Geometry: final body of the model. Coordinates: model frame, mm. Face numbers are marked on the shaded views. A direction names the side the tool comes from. Give positions to 0.01 mm unless a question says otherwise; leave off trailing zeros. Write each loop counter-clockwise with the first axis right and the second up, starting at its lowest first coordinate (ties: lowest second). Pieces come first, ordered by that corner, then holes. Notation, with made-up numbers: M -38,89.5 L -15,89.5 A36 cw -15,128.5 Z; hole C 52,75 d2. An arc over 180 degrees is marked long. Answer as a JSON object with one key per item and string values.
Autodesk Inventor part; units mm, degrees
ref_plane "YZ Plane" through (0, 0, 0) normal (1, 0, 0) x (0, 1, 0)
ref_plane "XZ Plane" through (0, 0, 0) normal (0, 1, 0) x (-1, 0, 0)
ref_plane "XY Plane" through (0, 0, 0) normal (0, 0, 1) x (1, 0, 0)
sketch "Sketch1" plane through (0, 0, 0) normal (0, 1, 0) x (-1, 0, 0)
  line L0 (0, 0) -> (56, 0)
  line L1 (56, 0) -> (56, -50)
  line L2 (56, -50) -> (0, -50)
  line L3 (0, -50) -> (0, 0)
  line L4 (56.2, 0) -> (-0.2, 0)
  line L5 (-0.2, 0) -> (-0.2, -50)
  line L6 (-0.2, -50) -> (56.2, -50)
  line L7 (56.2, -50) -> (56.2, 0)
  line L8 (58.7, 2.5) -> (-2.7, 2.5)
  line L9 (-2.7, 2.5) -> (-2.7, -52.5)
  line L10 (-2.7, -52.5) -> (58.7, -52.5)
  line L11 (58.7, -52.5) -> (58.7, 2.5)
  line L12 (56.2, -48.0985) -> (56.2, -52.5)
  line L13 (-0.2, -48.7936) -> (-0.2, -52.5)
  point P0 (-0.2, -50)
  dimension "d0" = 56
  dimension "d1" = 50
  dimension "d2" = 0.2
  dimension "d3" = 0.2
  dimension "d4" = 0
  dimension "d5" = 0
  dimension "d6" = 2.5
  dimension "d7" = 2.5
  dimension "d8" = 2.5
  dimension "d9" = 2.5
extrude "Extrusion1" add sketch "Sketch1" along normal blind 15.2 contours L4 L5 L13 L10 L9 L8 L11 L12 L7 L0
extrude "Extrusion2" add sketch "Sketch1" along normal blind 1
sketch "Sketch2" plane through (0.2, 15.2, 0) normal (0, 0, -1) x (-1, 0, 0)
  line L0 (0, -14.2) -> (0, 0)
  line L1 (0, -11.7) -> (56.4, -11.7)
  line L2 (56.4, -11.7) -> (56.4, -14.2)
  line L3 (56.4, -14.2) -> (0, -14.2)
  line L4 (0, -14.2) -> (0, -11.7)
  line L5 (56.4, -14.2) -> (56.4, 0)
  line L6 (0, -14.2) -> (56.4, -14.2)
  line L7 (1, -11.7) -> (55.4, -11.7)
  line L8 (55.4, -11.7) -> (55.4, -14.2)
  line L9 (55.4, -14.2) -> (1, -14.2)
  line L10 (1, -14.2) -> (1, -11.7)
  line L11 (0, -9) -> (56.4, -9)
  line L12 (56.4, -9) -> (56.4, -10)
  line L13 (56.4, -10) -> (0, -10)
  line L14 (0, -10) -> (0, -9)
  line L15 (56.4, -9) -> (55.4, -9)
  line L16 (55.4, -9) -> (55.4, -10)
  line L17 (55.4, -10) -> (56.4, -10)
  line L18 (56.4, -10) -> (56.4, -9)
  line L19 (0, -9) -> (1, -9)
  line L20 (1, -9) -> (1, -10)
  line L21 (1, -10) -> (0, -10)
  line L22 (0, -10) -> (0, -9)
  point P0 (0.2, -15.2)
  point P1 (0, -10)
  point P2 (1, -14.2)
  dimension "d14" = 0
  dimension "d16" = 2.5
  dimension "d17" = 1
  dimension "d18" = 1
  dimension "d19" = 0
  dimension "d20" = 0
  dimension "d21" = 1.7
  dimension "d22" = 1
extrude "Extrusion3" add sketch "Sketch2" along normal up to surface (52.5 mm away) contours L0 L1 L10 L3 | L0 L11 L20 L13 | L8 L1 L2 L3 | L16 L11 L5 L13
sketch "Sketch3" plane through (2.7, 0, -52.5) normal (0, 0, -1) x (-1, 0, 0)
  line L0 (2.5, 15.2) -> (58.9, 15.2)
  line L1 (23.5, 15.2) -> (43.9, 15.2)
  line L2 (43.9, 15.2) -> (43.9, 0)
  line L3 (43.9, 0) -> (23.5, 0)
  line L4 (23.5, 0) -> (23.5, 15.2)
  line L5 (58.9, 6.2) -> (58.9, 15.2)
  line L6 (2.5, 6.2) -> (2.5, 15.2)
  line L7 (0, 0) -> (61.4, 0)
  line L8 (23.5, 0) -> (43.9, 0)
  line L9 (43.9, 0) -> (43.9, 5)
  line L10 (43.9, 5) -> (23.5, 5)
  line L11 (23.5, 5) -> (23.5, 0)
  point P0 (2.7, 0)
  dimension "d25" = 15
  dimension "d26" = 21
  dimension "d27" = 0
  dimension "d30" = 5
extrude "Extrusion5" cut sketch "Sketch3" against normal blind 75.725 contours L10 L2 L3 L4
sketch "Sketch4" plane through (-58.7, 15.2, 2.5) normal (0, 0, 1) x (1, 0, 0)
  line L0 (11.5, -0.7) -> (20.5, -0.7)
  line L1 (20.5, -0.7) -> (20.5, -4.2)
  line L2 (20.5, -4.2) -> (11.5, -4.2)
  line L3 (11.5, -4.2) -> (11.5, -0.7)
  point P0 (58.7, -15.2)
  point P1 (3.5, -11.7)
  point P2 (2.5, -11.7)
  dimension "d33" = 7.5
  dimension "d34" = 11
  dimension "d35" = 18
  dimension "d36" = 9
extrude "Extrusion6" cut sketch "Sketch4" against normal up to surface (2.5 mm away)
sketch "Sketch5" plane through (0, 15.2, 0) normal (0, 1, 0) x (1, 0, 0)
  line L0 (2.7, -2.5) -> (2.7, 52.5)
  line L1 (2.7, -2.5) -> (2.7, 52.5)
  line L2 (2.7, 52.5) -> (0.2, 52.5)
  line L3 (2.7, 52.5) -> (0.2, 52.5)
  line L4 (0.2, 52.5) -> (0.2, 0)
  line L5 (0.2, 0) -> (-56.2, 0)
  line L6 (0.2, 0) -> (-56.2, 0)
  line L7 (-56.2, 52.5) -> (-58.7, 52.5)
  line L8 (-56.2, 0) -> (-56.2, 52.5)
  line L9 (-58.7, 52.5) -> (-58.7, -2.5)
  line L10 (-56.2, 52.5) -> (-58.7, 52.5)
  line L11 (-58.7, -2.5) -> (2.7, -2.5)
  line L12 (-58.7, 52.5) -> (-58.7, -2.5)
  line L13 (-58.7, -2.5) -> (2.7, -2.5)
  point P0 (0, 0)
extrude "Extrusion7" add sketch "Sketch5" along normal blind 3
sketch "Sketch6" plane through (0, 18.2, 0) normal (0, 1, 0) x (1, 0, 0)
  line L0 (2.7, -2.5) -> (2.7, 52.5)
  line L1 (-58.7, 52.5) -> (-58.7, -2.5)
  line L2 (2.7, -2.5) -> (-58.7, -2.5)
  line L3 (-58.7, -2.5) -> (-58.7, 52.5)
  line L4 (-58.7, 52.5) -> (2.7, 52.5)
  line L5 (2.7, 52.5) -> (2.7, -2.5)
  line L6 (-13.8, 42) -> (-1.8, 42)
  line L7 (-1.8, 42) -> (-1.8, 36)
  line L8 (-1.8, 36) -> (-13.8, 36)
  line L9 (-13.8, 36) -> (-13.8, 42)
  line L10 (0.2, 0) -> (-56.2, 0)
  line L11 (0.2, 52.5) -> (0.2, 0)
  line L12 (-10.8, 45) -> (-4.8, 45)
  line L13 (-13.8, 42) -> (-8.427, 47.373)
  line L14 (-13.8, 42) -> (-6.2015, 42) construction
  line L15 (-1.8, 42) -> (-7.8, 48)
  line L16 (-1.8, 42) -> (6.6853, 42) construction
  point P0 (0, 0)
  point P1 (-4.8, 45)
  point P2 (-58.7, -2.5)
  dimension "d41" = 36
  dimension "d42" = 42
  dimension "d43" = 2
  dimension "d44" = 14
  dimension "d45" = 3
  dimension "d46" = 3
  dimension "d47" = 45
  dimension "d48" = 135
  dimension "d49" = 3
extrude "Extrusion8" add sketch "Sketch6" along normal blind 1
sketch "Sketch7" plane through (2.7, 0, -52.5) normal (0, 0, -1) x (-1, 0, 0)
  line L0 (2.5, 3.5) -> (2.5, 5.2)
  line L1 (2.5, 3.5) -> (1.5, 3.5)
  line L2 (1.5, 3.5) -> (1.5, 5.2)
  line L3 (1.5, 5.2) -> (2.5, 5.2)
  line L4 (2.5, 5.2) -> (2.5, 3.5)
  line L5 (2.5, 6.2) -> (2.5, 18.2)
  line L6 (2.5, 18.2) -> (1.5, 18.2)
  line L7 (1.5, 18.2) -> (1.5, 6.2)
  line L8 (1.5, 6.2) -> (2.5, 6.2)
  line L9 (2.5, 6.2) -> (2.5, 18.2)
  line L10 (58.9, 3.5) -> (58.9, 5.2)
  line L11 (58.9, 3.5) -> (59.9, 3.5)
  line L12 (59.9, 3.5) -> (59.9, 5.2)
  line L13 (59.9, 5.2) -> (58.9, 5.2)
  line L14 (58.9, 5.2) -> (58.9, 3.5)
  line L15 (57.9, 6.2) -> (58.9, 6.2)
  line L16 (58.9, 6.2) -> (59.9, 6.2)
  line L17 (59.9, 6.2) -> (59.9, 18.2)
  line L18 (59.9, 18.2) -> (58.9, 18.2)
  line L19 (58.9, 18.2) -> (58.9, 6.2)
  point P0 (2.7, 0)
  dimension "d52" = 1
  dimension "d53" = 1
  dimension "d54" = 1
  dimension "d55" = 1
extrude "Extrusion9" cut sketch "Sketch7" against normal up to surface (52.5 mm away)
sketch "Sketch8" plane through (0, 19.2, 0) normal (0, 1, 0) x (1, 0, 0)
  line L0 (2.7, 52.5) -> (-20.8, 52.5)
  line L1 (-58.7, 52.5) -> (-58.7, -2.5)
  line L2 (2.7, 52.5) -> (-58.7, 52.5)
  line L3 (-58.7, 52.5) -> (-58.7, 49.5)
  line L4 (-58.7, 49.5) -> (2.7, 49.5)
  line L5 (2.7, 49.5) -> (2.7, 52.5)
  point P0 (0, 0)
  dimension "d58" = 3
extrude "Extrusion10" cut sketch "Sketch8" against normal up to surface (19.2 mm away)
sketch "Sketch9" plane through (0, 19.2, 0) normal (0, 1, 0) x (1, 0, 0)
  line L0 (2.7, -2.5) -> (2.7, 49.5)
  line L1 (-58.7, 49.5) -> (-58.7, -2.5)
  line L2 (2.7, 49.5) -> (-58.7, 49.5)
  line L3 (-58.7, 49.5) -> (-58.7, -2.5)
  line L4 (-58.7, -2.5) -> (2.7, -2.5)
  line L5 (2.7, -2.5) -> (2.7, 49.5)
  line L6 (-1.8, 42) -> (-1.8, 36)
  line L7 (-4.8, 45) -> (-1.8, 42)
  line L8 (-1.8, 42) -> (-4.8, 45)
  line L9 (-10.8, 45) -> (-4.8, 45)
  line L10 (-4.8, 45) -> (-10.8, 45)
  line L11 (-13.8, 42) -> (-10.8, 45)
  line L12 (-10.8, 45) -> (-13.8, 42)
  line L13 (-13.8, 36) -> (-13.8, 42)
  line L14 (-13.8, 42) -> (-13.8, 36)
  line L15 (-1.8, 36) -> (-13.8, 36)
  line L16 (-13.8, 36) -> (-1.8, 36)
  line L17 (-1.8, 36) -> (-1.8, 42)
  point P0 (0, 0)
extrude "Extrusion11" add sketch "Sketch9" along normal blind 1
sketch "Sketch10" plane through (1.2, 18.2, -49.5) normal (0, 0, -1) x (-1, 0, 0)
  line L0 (0, 0) -> (58.4, 0)
  line L1 (0, 0) -> (58.4, 0)
  line L2 (58.4, 0) -> (58.4, 1)
  line L3 (58.4, 1) -> (0, 1)
  line L4 (0, 1) -> (0, 0)
  point P0 (1.2, -18.2)
  dimension "d63" = 1
extrude "Extrusion12" cut sketch "Sketch10" against normal up to surface (49.5 mm away)
sketch "Sketch11" plane through (0, 20.2, 0) normal (0, 1, 0) x (1, 0, 0)
  line L0 (2.7, -2.5) -> (2.7, 49.5)
  line L1 (-58.7, 49.5) -> (-58.7, -2.5)
  line L2 (2.7, -2.5) -> (-58.7, -2.5)
  line L3 (-58.7, -2.5) -> (-58.7, -1)
  line L4 (-58.7, -1) -> (2.7, -1)
  line L5 (2.7, -1) -> (2.7, -2.5)
  point P0 (0, 0)
  dimension "d66" = 1.5
extrude "Extrusion13" cut sketch "Sketch11" against normal blind 24.925
sketch "Sketch12" plane through (-58.7, 20.2, 1) normal (0, 0, 1) x (1, 0, 0)
  line L0 (10.5, -3.7) -> (22.5, -3.7)
  line L1 (22.5, -3.7) -> (22.5, -11.2)
  line L2 (22.5, -11.2) -> (10.5, -11.2)
  line L3 (10.5, -11.2) -> (10.5, -3.7)
  line L4 (20.5, -5.7) -> (11.5, -5.7)
  line L5 (20.5, -9.2) -> (20.5, -5.7)
  line L6 (11.5, -9.2) -> (20.5, -9.2)
  line L7 (11.5, -5.7) -> (11.5, -9.2)
  point P0 (58.7, -20.2)
  dimension "d69" = 2
  dimension "d70" = 2
  dimension "d71" = 2
  dimension "d73" = 1
extrude "Extrusion14" cut sketch "Sketch12" against normal up to surface (1 mm away)
sketch "Sketch13" plane through (-58.7, 20.2, 1) normal (0, 0, 1) x (1, 0, 0)
  line L0 (29, 2.5) -> (41.7, 2.5)
  line L1 (41.7, 2.5) -> (41.7, 0)
  line L2 (41.7, 0) -> (19.7, 0)
  line L3 (19.7, 0) -> (19.7, 2.5)
  line L4 (0, 0) -> (61.4, 0)
  line L5 (0, -20.2) -> (0, 0)
  line L6 (16.7125, 7.282) -> (44.6875, 7.282)
  line L7 (44.6875, 7.282) -> (44.6875, 2.5)
  line L8 (16.7125, 2.5) -> (16.7125, 7.282)
  line L9 (29, 7.282) -> (32.4, 7.282)
  line L10 (32.4, 7.282) -> (32.4, 4.832)
  line L11 (32.4, 4.832) -> (29, 4.832)
  line L12 (29, 4.832) -> (29, 7.282)
  line L13 (44.6875, 2.5) -> (41.7, 2.5)
  line L14 (19.7, 2.5) -> (16.7125, 2.5)
  point P0 (58.7, -20.2)
  dimension "d76" = 0
  dimension "d77" = 2.5
  dimension "d78" = 22
  dimension "d79" = 61.4
  dimension "d80" = 19.7
  dimension "d81" = 4.782
  dimension "d83" = 27.975
  dimension "d84" = 16.7125
  dimension "d85" = 2.45
  dimension "d86" = 3.4
  dimension "d87" = 0
  dimension "d88" = 29
extrude "Extrusion15" add sketch "Sketch13" against normal blind 20 contours L1 L2 L3 L14 L8 L6 L12 L11 L10 L7 L13
sketch "Sketch14" plane through (-58.7, 20.2, -19) normal (0, 0, -1) x (-1, 0, 0)
  line L0 (-44.6875, 2.5) -> (-44.6875, 7.282)
  line L1 (-44.6875, 7.282) -> (-16.7125, 7.282)
  line L2 (-16.7125, 7.282) -> (-16.7125, 0)
  line L3 (-16.7125, 0) -> (-44.6875, 0)
  line L4 (-44.6875, 0) -> (-44.6875, 7.282)
  line L5 (-61.4, 0) -> (0, 0)
  line L6 (-16.7125, 2.5) -> (-16.7125, 7.282)
  point P0 (-58.7, -20.2)
  dimension "d91" = 0
  dimension "d92" = 0
extrude "Extrusion16" add sketch "Sketch14" along normal blind 1
chamfer "Chamfer1" distance 2.987 angle 45 2 edges at (-41.9875, 25.091, 1) (-14.0125, 25.091, 1)
chamfer "Chamfer2" distance 7.282 angle 45 1 edges at (-28, 20.2, -20)
equation "\"d23\" = d16"
properties part number "case+gopro"
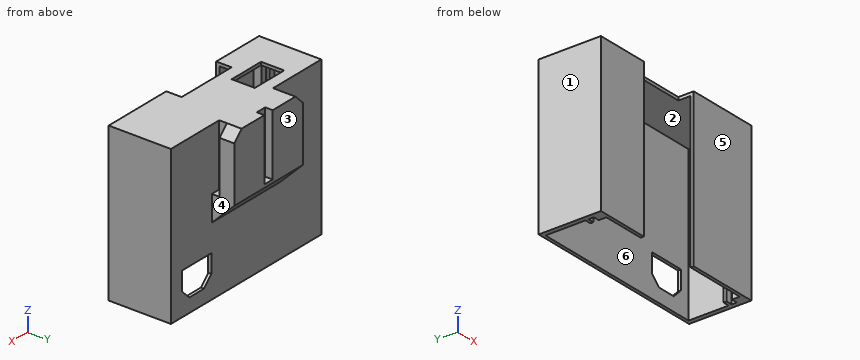
1) Pull-direction query (X, two-part tool) for the marked faces 1, 2 and 3; classes: pulls with the +X half, pulls with the -X half, needs draft (parallel to the pull), parting line crosses it, or undercut.
Geometry check:
{"face 1": "pulls with the -X half", "face 2": "undercut", "face 3": "needs draft"}
2) Set-up query: the marked faces 4, 5 and 6. Return all of +Z, -Z, +X, -X, +Y, -Y with unobstructed straight access to the full face (end or side cutting, diameter ignored); none if empty.
Geometry check:
{"face 4": "+Z, -Z, +X, +Y", "face 5": "+Z, -Z, +X, -X, -Y", "face 6": "-Z"}
3) Line query: line 1 (X direction, y = 4.75, z = -27); line 2 (X direction, y = 2, z = -22); line 3 (Y direction, x = -45.5, z = -14). Output: solid intervals per line, ascending. Write a range as from..to.
Geometry check:
{"line 1": "x = -58.7..-57.2, 1.2..2.7", "line 2": "x = -58.7..-55.2, -0.8..2.7", "line 3": "y = 0..1, 19.2..20.2"}
4) Cut plane B-B on z = -43.5. Return loops of the section in (x, y).
Geometry check:
{"outline": "M -58.7,0 L -41.2,0 L -41.2,1 L -55.2,1 L -55.2,3.5 L -57.2,3.5 L -57.2,5.2 L -55.2,5.2 L -55.2,6.2 L -57.2,6.2 L -57.2,19.2 L -12.3,19.2 L -12.3,20.2 L -58.7,20.2 Z; M -20.8,0 L 2.7,0 L 2.7,20.2 L -3.3,20.2 L -3.3,19.2 L 1.2,19.2 L 1.2,6.2 L -0.8,6.2 L -0.8,5.2 L 1.2,5.2 L 1.2,3.5 L -0.8,3.5 L -0.8,1 L -20.8,1 Z"}
5) Contact query for flat-ended pins moving along their axis: P1, Ø1.2, axis at y = 21, z = -6.5, coming from the -X side; P2, Ø3.5, axis at y = 23, z = -15, coming from the -X side; P3, Ø4, axis at x = -47.5, z = -16.5, coming from the +Y side; P4, Ø4, axis at x = -47, y = 23, coming from the -Z side. Output: stop coordinate, or through.
Geometry check:
{"P1": "stops at x = -39", "P2": "stops at x = -41.99", "P3": "stops at y = 20.2", "P4": "passes through"}
6) Cut plane A-A on x = -43. Return loops of the section in (y, z).
Geometry check:
{"outline": "M 0,-49.5 L 1,-49.5 L 1,0 L 9,0 L 9,1 L 0,1 Z; M 16.5,0 L 19.2,0 L 19.2,-49.5 L 20.2,-49.5 L 20.2,1 L 16.5,1 Z"}
7) Cut plane C-C on y = 10. Return loops of the section in (x, z), and give its area (3 significant figures).
Geometry check:
{"outline": "M -58.7,-49.5 L -57.2,-49.5 L -57.2,0 L -48.2,0 L -48.2,1 L -58.7,1 Z; M -36.2,0 L 1.2,0 L 1.2,-49.5 L 2.7,-49.5 L 2.7,1 L -36.2,1 Z", "area": "198 mm2"}
